from build123d import *

# Parameters (mm, degrees)
F1_DEPTH  = 80
F2_R      = 4
F3_DEPTH  = 8.5
F4_DEPTH  = 23.5
F5_R      = 15
F6_DEPTH  = 7
F7_R      = 15
F8_DEPTH  = 7
F9_R      = 5
F10_R     = 3.5
F11_DEPTH = 25
F13_DEPTH = 23.501
F15_DEPTH = 3
F16_R     = 11
F16_R_2   = 10
F17_DEPTH = 1
F18_R     = 11
F18_R_2   = 10
F19_DEPTH = 1
F20_R     = 3.5
F21_DEPTH = 32.001


with BuildPart() as f1:
    # F0 (on Front) → F1 (new body)
    with BuildSketch(Plane.XZ):
        with BuildLine():
            Line((0, 43), (0, 1))
            ThreePointArc((0, 1), (0.292893, 0.292893), (1, 0))
            Line((1, 0), (14, 0))
            ThreePointArc((14, 0), (14.707107, 0.292893), (15, 1))
            Line((15, 1), (15, 43))
            Line((15, 43), (12.5, 43))
            Line((12.5, 43), (12.5, 2.5))
            Line((12.5, 2.5), (2.5, 2.5))
            Line((2.5, 2.5), (2.5, 43))
            Line((2.5, 43), (0, 43))
        make_face()
    extrude(amount=F1_DEPTH)

    # F2 (on face) → F3 (join)
    with BuildSketch(Plane.YZ.offset(15)):
        with Locations((-60, 28)):
            Circle(F2_R)
        with Locations((-20, 28)):
            Circle(F2_R)
    extrude(amount=F3_DEPTH)

    # F2 (on face) → F4 (join)
    with BuildSketch(Plane.YZ.offset(15)):
        with Locations((-60, 28)):
            Circle(F2_R)
        with Locations((-20, 28)):
            Circle(F2_R)
    extrude(amount=-F4_DEPTH)

    # F5 (on face) → F6 (join)
    with BuildSketch(Plane.YZ.offset(23.5)):
        with Locations((-20, 28)):
            Circle(F5_R)
        with Locations((-60, 28)):
            Circle(F5_R)
    extrude(amount=-F6_DEPTH)

    # F7 (on face) → F8 (join)
    with BuildSketch(Plane(origin=(-8.5, 0, 0), x_dir=(0, -1, 0), z_dir=(-1, 0, 0))):
        with Locations((20, 28)):
            Circle(F7_R)
        with Locations((60, 28)):
            Circle(F7_R)
    extrude(amount=-F8_DEPTH)

    # F9
    f9_edges = [f1.edges().sort_by_distance(p)[0] for p in [
        (1.25, -80, 43),
        (13.75, -80, 43),
        (1.25, 0, 43),
        (13.75, 0, 43),
    ]]
    fillet(f9_edges, radius=F9_R)

    # F10 (on face) → F11 (cut)
    with BuildSketch(Plane(origin=(0, 0, 0), x_dir=(1, 0, 0), z_dir=(0, 0, -1))):
        with Locations((7.5, 40)):
            Circle(F10_R)
    extrude(amount=-F11_DEPTH, mode=Mode.SUBTRACT)

    # F12 (on face) → F13 (cut, through all)
    with BuildSketch(Plane.YZ.offset(15)):
        with BuildLine():
            ThreePointArc((-29.5, 2.5), (-28.085786, 3.085786), (-27.5, 4.5))
            Line((-27.5, 4.5), (-27.5, 10.5))
            ThreePointArc((-27.5, 10.5), (-28.085786, 11.914214), (-29.5, 12.5))
            Line((-29.5, 12.5), (-50.5, 12.5))
            ThreePointArc((-50.5, 12.5), (-51.914214, 11.914214), (-52.5, 10.5))
            Line((-52.5, 10.5), (-52.5, 4.5))
            ThreePointArc((-52.5, 4.5), (-51.914214, 3.085786), (-50.5, 2.5))
            Line((-50.5, 2.5), (-29.5, 2.5))
        make_face()
    extrude(amount=-F13_DEPTH, mode=Mode.SUBTRACT)

    # F14 (on face) → F15 (cut)
    with BuildSketch(Plane(origin=(0, 0, 0), x_dir=(1, 0, 0), z_dir=(0, 0, -1))):
        with BuildLine():
            Line((10, 70), (7.5, 70))
            Line((7.5, 70), (5, 70))
            ThreePointArc((5, 70), (4.292893, 69.707107), (4, 69))
            Line((4, 69), (4, 57))
            ThreePointArc((4, 57), (4.292893, 56.292893), (5, 56))
            Line((5, 56), (10, 56))
            ThreePointArc((10, 56), (10.707107, 56.292893), (11, 57))
            Line((11, 57), (11, 69))
            ThreePointArc((11, 69), (10.707107, 69.707107), (10, 70))
        make_face()
        with BuildLine():
            ThreePointArc((10, 10), (10.707107, 10.292893), (11, 11))
            Line((11, 11), (11, 23))
            ThreePointArc((11, 23), (10.707107, 23.707107), (10, 24))
            Line((10, 24), (5, 24))
            ThreePointArc((5, 24), (4.292893, 23.707107), (4, 23))
            Line((4, 23), (4, 11))
            ThreePointArc((4, 11), (4.292893, 10.292893), (5, 10))
            Line((5, 10), (7.5, 10))
            Line((7.5, 10), (10, 10))
        make_face()
    extrude(amount=-F15_DEPTH, mode=Mode.SUBTRACT)

    # F16 (on face) → F17 (cut)
    with BuildSketch(Plane(origin=(-8.5, 0, 0), x_dir=(0, -1, 0), z_dir=(-1, 0, 0))):
        with Locations((20, 28)):
            Circle(F16_R)
        with Locations((20, 28)):
            Circle(F16_R_2, mode=Mode.SUBTRACT)
        with Locations((60, 28)):
            Circle(F16_R)
        with Locations((60, 28)):
            Circle(F16_R_2, mode=Mode.SUBTRACT)
    extrude(amount=-F17_DEPTH, mode=Mode.SUBTRACT)

    # F18 (on face) → F19 (cut)
    with BuildSketch(Plane.YZ.offset(23.5)):
        with Locations((-60, 28)):
            Circle(F18_R)
        with Locations((-60, 28)):
            Circle(F18_R_2, mode=Mode.SUBTRACT)
        with Locations((-20, 28)):
            Circle(F18_R)
        with Locations((-20, 28)):
            Circle(F18_R_2, mode=Mode.SUBTRACT)
    extrude(amount=-F19_DEPTH, mode=Mode.SUBTRACT)

    # F20 (on face) → F21 (cut, through all)
    with BuildSketch(Plane.YZ.offset(23.5)):
        with Locations((-20, 28)):
            Circle(F20_R)
        with Locations((-60, 28)):
            Circle(F20_R)
    extrude(amount=-F21_DEPTH, mode=Mode.SUBTRACT)


solid = f1.part
Build history of the part. All positions in model axes, mm. A direction names the side the tool comes from. Give positions to 0.01 mm unless a question says otherwise; leave off trailing zeros. Loops run counter-clockwise (first coordinate to the right, second up) from the corner with the lowest first, then second, coordinate; pieces in that order, holes last. Notation, with made-up numbers: (-9.75, 62.25) - (42.25, 62.25) arc R15 cw to (42.25, 78.25) - close; hole circle Ø2 at (51.25, 54.25). An arc over 180 degrees is marked (long way). Write item = value, one per line. Start each with the question number.
1) Tool access for faces 5 (the flat face through (3, -41, 2.5)), 6 (the flat face through (7, -56, 1)), 7 (the cylindrical face through (23.007, -14.924, 18.241)), 8 (the cylindrical face through (-5.049, -16.748, 13.357)), 9 (the cylindrical face through (1.27, -28.07, 11.9)): list every direction of +Z, -Z, +X, -X, +Y, -Y with a clear straight run to the whole face (end or side of a thin tool).
2) Band-saw the part on A-A on y = -40. Give the cut face in (x, z), plus the area to 3 significant figures.
3) Band-saw the part on D-D on y = -72.5. Give the cut face in (x, z).
4) Band-saw the part on C-C on x = 7. Give the cut face in (y, z), plus the area to 3 significant figures.
5) Probe probe 1 along X at (y, z) = (-63, 15); probe 2 along Z at (x, y) = (23.2, -60); probe 3 along Z at (x, y) = (16, -20). List the from-to ranges inside material, lowest first. Write a range as from..to.
6) Band-saw the part on B-B on z = 16. Give the cut face in (x, y).
7) Pull direction Z, two halves, no side cores. Call faces 1 (the cylindrical face through (15.74, -20.521, 31.966)), 2 (the cylindrical face through (1.27, -51.9, 11.93)), 3 (the flat face through (16.5, -57, 25)), 4 (the cylindrical face through (-8.007, -24.614, 19.128)): +Z half, -Z half, draft (parallel to the pull), parting line (faces both ways), or undercut.
8) Drop flat-ended pins along their axis: pin 1 Ø8 at (y, z) = (-42.5, 9.5) entering from +X; pin 2 Ø12 at (y, z) = (-69, 7.5) entering from -X. Give the stop position or say it passes through.
Final values:
q1.face_5 = none
q1.face_6 = -Z
q1.face_7 = +X
q1.face_8 = -X
q1.face_9 = +X, -X
q2.outline = (0, 1) arc R1 ccw to (1, 0) - (4, 0) - (4, 2.5) - (0, 2.5) - close; (0, 12.5) - (2.5, 12.5) - (2.5, 43) - (0, 43) - close; (11, 0) - (14, 0) arc R1 ccw to (15, 1) - (15, 2.5) - (11, 2.5) - close; (12.5, 12.5) - (15, 12.5) - (15, 43) - (12.5, 43) - close
q2.area = 172 mm²
q3.outline = (-8.5, 19.71) - (-1.5, 19.71) - (-1.5, 36.29) - (-8.5, 36.29) - close; (0, 1) arc R1 ccw to (1, 0) - (14, 0) arc R1 ccw to (15, 1) - (15, 43) - (12.5, 43) - (12.5, 2.5) - (2.5, 2.5) - (2.5, 43) - (0, 43) - close; (16.5, 19.71) - (23.5, 19.71) - (23.5, 36.29) - (16.5, 36.29) - close
q4.outline = (-80, 0) - (-70, 0) - (-70, 2.5) - (-80, 2.5) - close; circle Ø8 at (-60, 28); (-56, 0) - (-43.46, 0) - (-43.46, 2.5) - (-56, 2.5) - close; (-36.54, 0) - (-24, 0) - (-24, 2.5) - (-36.54, 2.5) - close; circle Ø8 at (-20, 28); (-10, 0) - (0, 0) - (0, 2.5) - (-10, 2.5) - close; hole circle Ø7 at (-60, 28); hole circle Ø7 at (-20, 28)
q4.area = 136 mm²
q5.probe_1 = -8.5..-1.5, 0..2.5, 12.5..15, 16.5..23.5
q5.probe_2 = 13..17, 18..24.5, 31.5..38, 39..43
q5.probe_3 = 24..24.5, 31.5..32
q6.outline = (-8.5, -69) - (-1.5, -69) - (-1.5, -51) - (-8.5, -51) - close; (-8.5, -29) - (-1.5, -29) - (-1.5, -11) - (-8.5, -11) - close; (0, -80) - (2.5, -80) - (2.5, 0) - (0, 0) - close; (12.5, -80) - (15, -80) - (15, 0) - (12.5, 0) - close; (16.5, -69) - (23.5, -69) - (23.5, -51) - (16.5, -51) - close; (16.5, -29) - (23.5, -29) - (23.5, -11) - (16.5, -11) - close
q7.face_1 = parting line
q7.face_2 = undercut
q7.face_3 = draft
q7.face_4 = undercut
q8.pin_1 = 15
q8.pin_2 = 0
